Check sheet for the modelled part. Datum: model origin and axes. Units: mm. Face numbers are marked on the shaded views. A direction names the side the tool comes from. Give positions to 0.01 mm unless a question says otherwise; leave off trailing zeros. Loops run counter-clockwise (first coordinate to the right, second up) from the corner with the lowest first, then second, coordinate; pieces in that order, holes last. Notation, with made-up numbers: (68.25, 60) -> (81.25, 60) arc R32 cw to (81.25, 96) -> close; hole circle Ø1 at (12, -38). An arc over 180 degrees is marked (long way). Answer as CSV lines item,"result". Start each with the question number.
(1) Section check D-D on y = 6.5. Enter the section's corners in (x, z).
(2) Access from +Z, -Z, +X, -X, +Y, -Y to the whole of each face (thin tool, end or side, straight path). Record for the marked faces 1, 2 and 3.
(3) Section check A-A on x = 0. Enter the section's corners in (y, z), plus the area to 3 significant figures.
(4) Release check for a two-part mould opening along X. For the marked faces 4, 5 and 6 record: pulls with the +X half, pulls with the -X half, needs draft (parallel to the pull), parting line crosses it, or undercut.
(5) Gauge pin test, flat ends, axial feed: pin 1 Ø4 at (y, z) = (-7, 6) entering from -X; pin 2 Ø1.2 at (y, z) = (2.5, -0.5) entering from +X; pin 3 Ø4 at (x, z) = (10, 2.5) entering from -Y; pin 4 Ø1.5 at (x, z) = (-9, 4) entering from -Y. Record the tip position at first contact, or that the pin passes through.
(6) Material ranges on line 1 (Y direction, x = 0, z = 4.55); line 2 (Z direction, x = 8, y = -8); line 3 (Y direction, x = 0, z = 0.45), recorded low to high. Write a range as from..to.
(7) Section check B-B on y = 13. Enter the section's corners in (x, z).
(8) Section check C-C on z = 3.75. Enter the section's corners in (x, y), plus the area to 3 significant figures.
from build123d import *

# Parameters (mm, degrees)
SKETCH_1_W            = 3
SKETCH_1_H            = 1
CUT_EXTRUDE_START     = 0.339415
SKETCH_3_W            = 1.1
SKETCH_3_H            = 2.4
CUT_EXTRUDE_899_DEPTH = 4.668984
SKETCH_4_R            = 8
EXTRUDE_1_DEPTH       = 2
SKETCH_5_R            = 2.5
EXTRUDE_2_DEPTH       = 3
CUT_EXTRUDE_2_REACH   = 30.671


with BuildPart() as part:
    # 草图1 → Revolve 702 (revolve)
    with BuildSketch(Plane(origin=(0, 0, 0), x_dir=(0, 0, -1), z_dir=(1, 0, 0)), mode=Mode.PRIVATE) as revolve_702_sk:
        Polygon((1.5, 7), (1.5, 6), (2.5, 6), (2.5, 19), (1.5, 19), align=None)
        with Locations((0, 6.5)):
            Rectangle(SKETCH_1_W, SKETCH_1_H)
        Polygon((-2.5, 6), (-1.5, 6), (-1.5, 7), (-1.5, 19), (-2.5, 19), align=None)
    revolve(revolve_702_sk.sketch.rotate(Axis((0, 0, 1.65), (0, 0, -1)), 90), axis=Axis((0, 0, 1.65), (0, 0, -1)))

    # 草图3 → Cut-Extrude 899 (cut)
    with BuildSketch(Plane(origin=(0, 0, 0), x_dir=(1, 0, 0), z_dir=(0, 1, 0)).offset(CUT_EXTRUDE_START)):
        with Locations((-5.440392091, 0)):
            Rectangle(SKETCH_3_W, SKETCH_3_H)
    extrude(amount=CUT_EXTRUDE_899_DEPTH, mode=Mode.SUBTRACT)

    # 草图4 → 凸台-拉伸1 (add)
    with BuildSketch(Plane.XY.offset(2.5)):
        Circle(SKETCH_4_R)
    extrude(amount=EXTRUDE_1_DEPTH)

    # 草图5 → 凸台-拉伸2 (add)
    with BuildSketch(Plane.XY.offset(4.5)):
        Circle(SKETCH_5_R)
    extrude(amount=EXTRUDE_2_DEPTH)

    # 草图6 → 切除-拉伸2 (cut, up to next)
    with BuildSketch(Plane.XY.offset(7.5), mode=Mode.PRIVATE) as cut_extrude_2_sk1:
        with BuildLine():
            Line((-1.174734012, -0.85), (1.174734012, -0.85))
            ThreePointArc((1.174734012, -0.85), (1.379468071, -0.446730166), (1.45, 0))
            ThreePointArc((1.45, 0), (-0.446730166, 1.379468071), (-1.174734012, -0.85))
        make_face()
    cut_extrude_2_tool1 = extrude(cut_extrude_2_sk1.sketch, amount=-CUT_EXTRUDE_2_REACH, mode=Mode.PRIVATE) & part.part
    add(cut_extrude_2_tool1.solids().sort_by_distance((0, 0.192371, 7.5))[0], mode=Mode.SUBTRACT)


solid = part.part
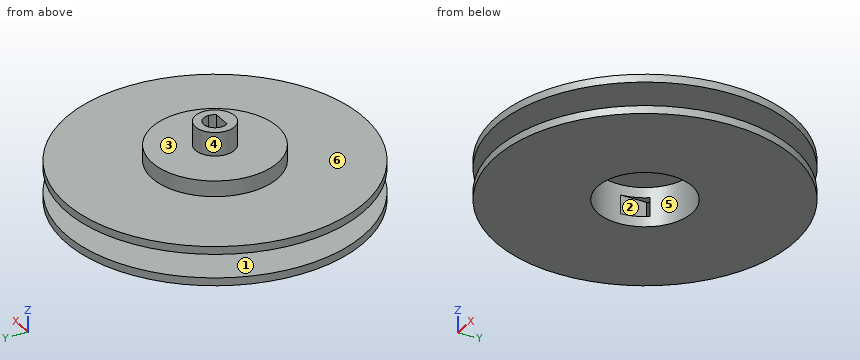
Working result:
1,outline,"(-17.85, -2.5) -> (17.85, -2.5) -> (17.85, -1.5) -> (2.6, -1.5) -> (2.6, 1.5) -> (17.85, 1.5) -> (17.85, 2.5) -> (4.66, 2.5) -> (4.66, 4.5) -> (-4.66, 4.5) -> (-4.66, 2.5) -> (-17.85, 2.5) -> (-17.85, 1.5) -> (-2.6, 1.5) -> (-2.6, -1.5) -> (-17.85, -1.5) -> close"
2,face 1,"none"
2,face 2,"+Y"
2,face 3,"+Z"
3,outline,"(-19, -2.5) -> (-6, -2.5) -> (-6, 2.5) -> (-0.85, 2.5) -> (-0.85, 7.5) -> (-2.5, 7.5) -> (-2.5, 4.5) -> (-8, 4.5) -> (-8, 2.5) -> (-19, 2.5) -> (-19, 1.5) -> (-7, 1.5) -> (-7, -1.5) -> (-19, -1.5) -> close; (1.45, 2.5) -> (6, 2.5) -> (6, -2.5) -> (19, -2.5) -> (19, -1.5) -> (7, -1.5) -> (7, 1.5) -> (19, 1.5) -> (19, 2.5) -> (8, 2.5) -> (8, 4.5) -> (2.5, 4.5) -> (2.5, 7.5) -> (1.45, 7.5) -> close"
3,area,"93.5 mm^2"
4,face 4,"parting line crosses it"
4,face 5,"undercut"
4,face 6,"needs draft"
5,pin 1,"stops at x = -5.64"
5,pin 2,"stops at x = 6.74"
5,pin 3,"stops at y = -17.23"
5,pin 4,"passes through"
6,line 1,"y = -2.5..-0.85, 1.45..2.5"
6,line 2,"z = -2.5..-1.5, 1.5..2.5"
6,line 3,"y = -7..-6, 6..7"
7,outline,"(-13.86, -2.5) -> (13.86, -2.5) -> (13.86, -1.5) -> (-13.86, -1.5) -> close; (-13.86, 1.5) -> (13.86, 1.5) -> (13.86, 2.5) -> (-13.86, 2.5) -> close"
8,outline,"circle Ø16 at (0, 0); hole (-1.17, -0.85) -> (1.17, -0.85) arc R1.45 ccw (long way) to start"
8,area,"195 mm^2"
